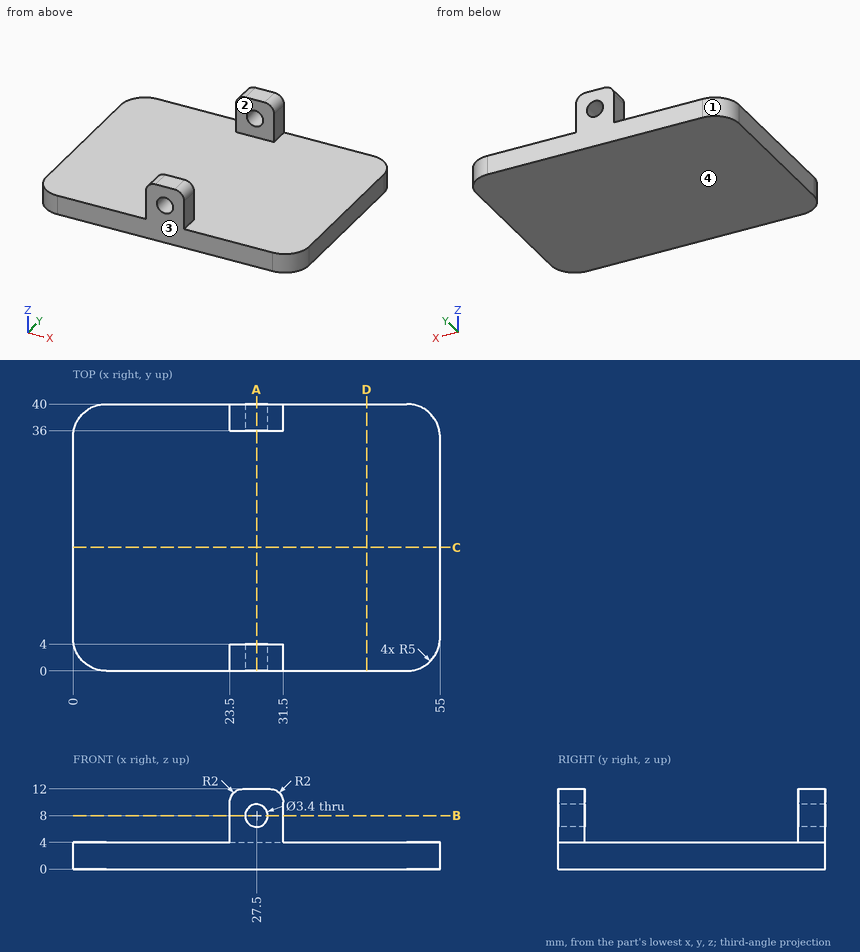
Part print with two shaded views. Sizes in mm from the minimum x, y, z corner. Coordinates: 2 decimals unless noted, no trailing zeros. Write each loop counter-clockwise with the first axis right and the second up, starting at its lowest first coordinate (ties: lowest second). Pieces come first, ordered by that corner, then holes. Notation, with made-up numbers: (48, 35.5) - (57, 35.5) arc R10 cw to (57, 44.5) - close; hole circle Ø7 at (1, 25). An arc over 180 degrees is marked (long way). Use a Markdown table: item, result. Add a question column.
Item 1: Drop flat-ended pins along their axis: pin 1 (10 mm diameter, centred on x = 29.5, y = 19, fed in from +Z); pin 2 (1.2 mm diameter, centred on y = 39, z = 6.5, fed in from -X); pin 3 (1.2 mm diameter, centred on y = 38.5, z = 7.5, fed in from +X). Give the stop position or say it passes through.
Item 2: Band-saw the part on C-C, the plane y = 18.5. Write the cut outline in (x, z).
Item 3: Two-plate mould, pull along Y, no slides. Class the marked faces 1, 2, 3 and 4: pulls with the +Y half, pulls with the -Y half, needs draft (parallel to the pull), parting line crosses it, or undercut.
Item 4: Band-saw the part on B-B, the plane z = 8. Write the cut outline in (x, y), and give its area (3 significant figures).
Item 5: Drill centre lines: line 1 along Z through (x, y) = (27.5, 1.3); line 2 along Y through (x, z) = (24.5, 10); line 3 along Z through (x, y) = (22, 4). Where is each one in solid material? Low to high.
Item 6: Band-saw the part on D-D, the plane x = 44. Write the cut outline in (y, z), and give its area (3 significant figures).
Item 7: Band-saw the part on A-A, the plane x = 27.5. Write the cut outline in (y, z).
A:
| question | item | result |
|---|---|---|
| 1 | pin 1 | stops at z = 4 |
| 1 | pin 2 | stops at x = 23.5 |
| 1 | pin 3 | stops at x = 31.5 |
| 2 | outline | (0, 0) - (55, 0) - (55, 4) - (0, 4) - close |
| 3 | face 1 | pulls with the +Y half |
| 3 | face 2 | undercut |
| 3 | face 3 | pulls with the -Y half |
| 3 | face 4 | needs draft |
| 4 | outline | (23.5, 0) - (25.8, 0) - (25.8, 4) - (23.5, 4) - close; (23.5, 36) - (25.8, 36) - (25.8, 40) - (23.5, 40) - close; (29.2, 0) - (31.5, 0) - (31.5, 4) - (29.2, 4) - close; (29.2, 36) - (31.5, 36) - (31.5, 40) - (29.2, 40) - close |
| 4 | area | 36.8 mm² |
| 5 | line 1 | z = 0 to 6.3, 9.7 to 12 |
| 5 | line 2 | y = 0 to 4, 36 to 40 |
| 5 | line 3 | z = 0 to 4 |
| 6 | outline | (0, 0) - (40, 0) - (40, 4) - (0, 4) - close |
| 6 | area | 160 mm² |
| 7 | outline | (0, 0) - (40, 0) - (40, 6.3) - (36, 6.3) - (36, 4) - (4, 4) - (4, 6.3) - (0, 6.3) - close; (0, 9.7) - (4, 9.7) - (4, 12) - (0, 12) - close; (36, 9.7) - (40, 9.7) - (40, 12) - (36, 12) - close |
